from build123d import *

# Parameters (mm, degrees)
CUT_EXTRUDE_START    = -17
CUT_EXTRUDE_1_DEPTH  = 1.580856159
EXTRUDE_1_REACH      = 29.331
EXTRUDE_1_END_RADIUS = 16
SKETCH_3_W           = 10
SKETCH_3_H           = 6
SKETCH_3_W_2         = 6.5
SKETCH_3_H_2         = 3.5
SKETCH_4_R           = 0.5


# Read off the part's stored shape, not the designer's step: 切除-拉伸1
with BuildPart() as part:
    # 草图1 → 旋转1 (revolve)
    with BuildSketch(Plane(origin=(0, 0, 0), x_dir=(1, 0, 0), z_dir=(0, 1, 0))):
        with BuildLine():
            Line((15.491933385, 4), (15.491933385, 0))
            Line((15.491933385, 0), (17, 0))
            ThreePointArc((17, 0), (12.02081528, 12.02081528), (0, 17))
            Line((0, 17), (0, 16))
            ThreePointArc((0, 16), (9.797958971, 12.649110641), (15.491933385, 4))
        make_face()
    revolve(axis=Axis((0, 0, -17), (0, 0, 1)))

    # 切除-拉伸1 outline → 切除-拉伸1 (cut)
    with BuildSketch(Plane(origin=(0, 0, 0), x_dir=(1, 0, 0), z_dir=(0, 1, 0)).offset(CUT_EXTRUDE_START)):
        with BuildLine():
            Line((-1.5, 0), (1.5, 0))
            ThreePointArc((1.5, 0), (0, 1.5), (-1.5, 0))
        make_face()
    extrude(amount=CUT_EXTRUDE_1_DEPTH, mode=Mode.SUBTRACT)

    # 凸台-拉伸1: up to this sphere (the profile starts inside it)
    extrude_1_end = Location((0, 0, 0)) * Sphere(EXTRUDE_1_END_RADIUS, mode=Mode.PRIVATE)
    # 草图3 → 凸台-拉伸1 (add, up to the surface)
    with BuildSketch(Plane.XY.offset(-4), mode=Mode.PRIVATE) as extrude_1_sk1:
        with Locations((0, -11)):
            Rectangle(SKETCH_3_W, SKETCH_3_H)
        with Locations((0, -11)):
            Rectangle(SKETCH_3_W_2, SKETCH_3_H_2, mode=Mode.SUBTRACT)
    extrude_1_tool1 = extrude(extrude_1_sk1.sketch, amount=-EXTRUDE_1_REACH, mode=Mode.PRIVATE) & extrude_1_end
    add(extrude_1_tool1.solids().sort_by_distance((0, -8.116619, -4))[0])

    # 草图4 → 切除-旋转1 (revolve, cut)
    with BuildSketch(Plane(origin=(0, 0, 0), x_dir=(1, 0, 0), z_dir=(0, 1, 0))):
        with Locations((9, 14.422205102)):
            Circle(SKETCH_4_R)
    revolve(axis=Axis((0, 0, 0), (0, 0, -1)), mode=Mode.SUBTRACT)


solid = part.part
Can you work these out from the model? Positions are in its coordinate system, mm. A direction names the side the tool comes from. Give positions to 0.01 mm unless a question says otherwise; leave off trailing zeros. Write each loop counter-clockwise with the first axis right and the second up, starting at its lowest first coordinate (ties: lowest second). Pieces come first, ordered by that corner, then holes. Notation, with made-up numbers: (-2, 43) -> (14, 43) arc R15 ccw to (14, 49) -> close; hole circle Ø3 at (-21, 32.25). An arc over 180 degrees is marked (long way). Answer as a JSON object with one key per item and string values. Group by question number.
Item 1: I'm going to push flat-ended pins straight in: P1, Ø3, axis at y = -2, z = -8.5, coming from the -X side; P2, Ø1.9, axis at x = 2, z = -6.5, coming from the -Y side; P3, Ø1.5, axis at y = 0, z = -6, coming from the -X side; P4, Ø10, axis at x = -1.5, z = -3, coming from the +Y side. Where does each tip first touch, or does it pass through?
Item 2: Please list where these lines run through material, in increasing order: line 1 (X direction, y = 0, z = -1.65); line 2 (X direction, y = 0, z = -2.85); line 3 (Y direction, x = 0, z = -2.75). Write a range as [from, to].
Item 3: Suppose I cut it at D-D (x = 12.5). Please give me the cut outline in (y, z).
Item 4: Suppose I cut it at A-A (z = -10.5). Please give me the cut outline in (x, y).
Item 5: For faces 1 (the face through (14.777, 4.653, -1.972)), 2 (the face through (0, -16.2, -1.5)), 3 (the face through (-14, -7, 0)), which set-ups out of +Z, -Z, +X, -X, +Y, -Y let a thin tool reach every point of the face, with its end or its side?
Item 6: Suppose I cut it at B-B (x = 0). Please give me the cut outline in (y, z), plus the area to 3 significant figures.
Item 7: Suppose I cut it at C-C (y = 0). Please give me the cut outline in (x, z).
Findings:
{
 "1": {"P1": "stops at x = -15.38", "P2": "stops at y = -15.96", "P3": "stops at x = -16.17", "P4": "stops at y = 17"},
 "2": {"line 1": "x = [-16.92, -15.49], [15.49, 16.92]", "line 2": "x = [-16.76, -15.49], [15.49, 16.76]", "line 3": "y = [-16.78, -15.49], [15.49, 16.78]"},
 "3": {"outline": "(-11.52, 0) arc R11.52 ccw to (11.52, 0) -> (9.15, 0) -> (9.15, -4) arc R9.99 cw to (-9.15, -4) -> (-9.15, 0) -> close"},
 "4": {"outline": "circle Ø26.74 at (0, 0); hole (-5, -10.99) -> (-5, -8) -> (5, -8) -> (5, -10.99) arc R12.07 ccw (long way) to start; hole (-3.25, -11.63) arc R12.07 ccw to (3.25, -11.63) -> (3.25, -9.25) -> (-3.25, -9.25) -> close"},
 "5": {"face 1": "+Z", "face 2": "+Z, -Y", "face 3": "+Z, +X, -X, +Y, -Y"},
 "6": {"outline": "(-16.93, -1.5) arc R17 ccw to (-9.42, -14.15) arc R0.5 cw to (-8.57, -14.68) arc R17 ccw to (8.57, -14.68) arc R0.5 cw to (9.42, -14.15) arc R17 ccw to (17, 0) -> (15.49, 0) -> (15.49, -4) arc R16 cw to (-8, -13.86) -> (-8, -4) -> (-9.25, -4) -> (-9.25, -13.06) arc R16 cw to (-12.75, -9.67) -> (-12.75, -4) -> (-14, -4) -> (-14, -7.75) arc R16 cw to (-15.49, -4) -> (-15.49, -1.5) -> close", "area": "69.3 mm²"},
 "7": {"outline": "(-17, 0) arc R17 ccw to (-9.42, -14.15) arc R0.5 cw to (-8.57, -14.68) arc R17 ccw to (8.57, -14.68) arc R0.5 cw to (9.42, -14.15) arc R17 ccw to (17, 0) -> (15.49, 0) -> (15.49, -4) arc R16 cw to (-15.49, -4) -> (-15.49, 0) -> close"}
}
